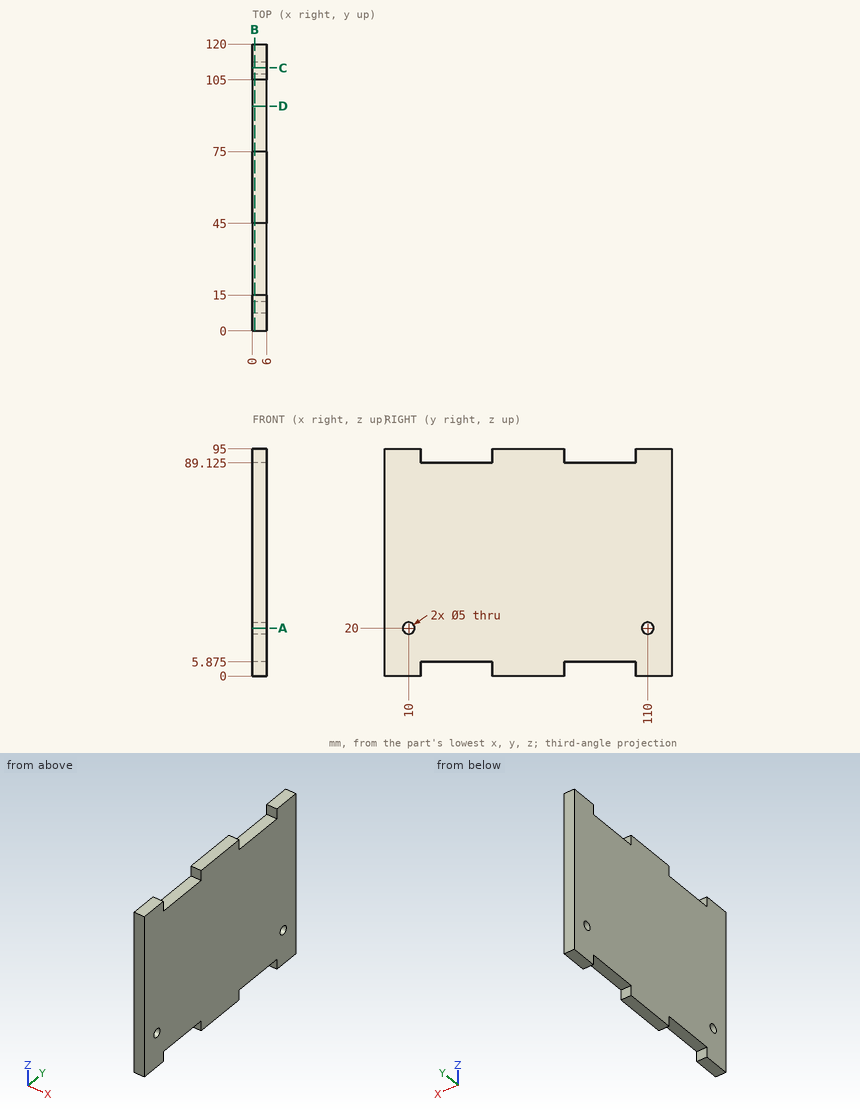
The figure shows three views and two pictorial views of one solid part (mm, origin at its lowest corner). Answer the questions. Coordinates: 2 decimals unless noted, no trailing zeros. Write each loop counter-clockwise with the first axis right and the second up, starting at its lowest first coordinate (ties: lowest second). Pieces come first, ordered by that corner, then holes. Notation, with made-up numbers: (40, 11.5) -> (80, 11.5) arc R4 cw to (80, 16.5) -> close; hole circle Ø11 at (48, 71). An arc over 180 degrees is marked (long way). Return JSON: item names as keys, results as strings.
1. A cutting plane is placed at C-C (y = 110). Determine the outline of the cut face in (x, z), and give its area (3 significant figures).
Found:
{"outline": "(0, 0) -> (6, 0) -> (6, 17.5) -> (0, 17.5) -> close; (0, 22.5) -> (6, 22.5) -> (6, 95) -> (0, 95) -> close", "area": "540 mm2"}
2. Find the intervals of material crossed by line 1 along Y through (x, z) = (2.65, 20); line 2 along Z through (x, y) = (1.25, 17) (3 decimals), in increasing order. Write a range as from..to.
Found:
{"line 1": "0..7.5, 12.5..107.5, 112.5..120", "line 2": "5.875..89.125"}
3. A cutting plane is placed at D-D (y = 94). Determine the outline of the cut face in (x, z) (3 decimals), and give its area (4 significant figures).
Found:
{"outline": "(0, 5.875) -> (6, 5.875) -> (6, 89.125) -> (0, 89.125) -> close", "area": "499.5 mm2"}
4. This flat-tipped pin is pushed along its axis until it touches: P1, Ø1.5, axis at x = 3, y = 39.5, coming from the +Z side (3 decimals). Where does it stop, or does it pass through?
Found:
{"P1": "z = 89.125"}
5. A cutting plane is placed at B-B (x = 0.9). Determine the outline of the cut face in (y, z) (3 decimals).
Found:
{"outline": "(0, 0) -> (15, 0) -> (15, 5.875) -> (45, 5.875) -> (45, 0) -> (75, 0) -> (75, 5.875) -> (105, 5.875) -> (105, 0) -> (120, 0) -> (120, 95) -> (105, 95) -> (105, 89.125) -> (75, 89.125) -> (75, 95) -> (45, 95) -> (45, 89.125) -> (15, 89.125) -> (15, 95) -> (0, 95) -> close; hole circle Ø5 at (10, 20); hole circle Ø5 at (110, 20)"}
6. A cutting plane is placed at A-A (z = 20). Determine the outline of the cut face in (x, y), and give its area (3 significant figures).
Found:
{"outline": "(0, 0) -> (6, 0) -> (6, 7.5) -> (0, 7.5) -> close; (0, 12.5) -> (6, 12.5) -> (6, 107.5) -> (0, 107.5) -> close; (0, 112.5) -> (6, 112.5) -> (6, 120) -> (0, 120) -> close", "area": "660 mm2"}
